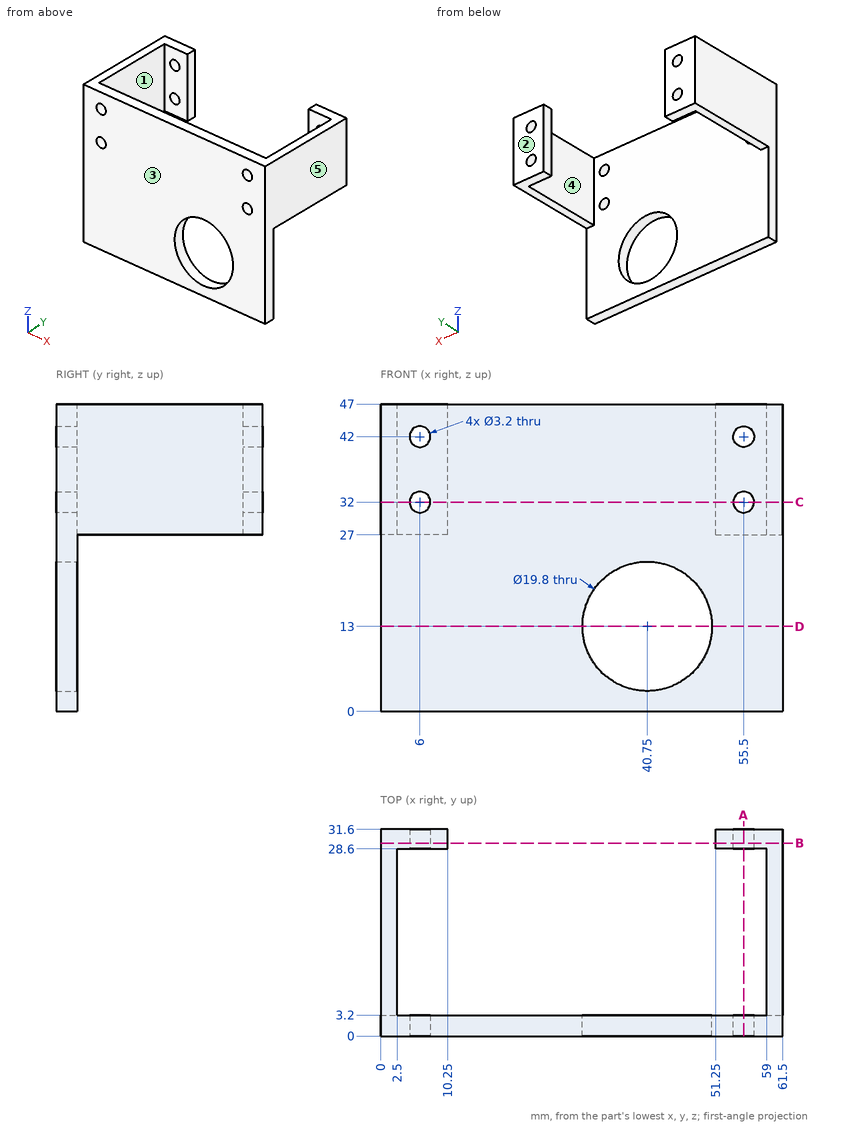
Source: three-view drawing plus pictorial views. Frame: mm from the lowest corner of the part. A direction names the side the tool comes from. Round coordinates to 2 decimals unless told otherwise and drop trailing zeros. Write each loop counter-clockwise with the first axis right and the second up, starting at its lowest first coordinate (ties: lowest second). Pieces come first, ordered by that corner, then holes. Notation, with made-up numbers: M -4.75,20.5 L 46.25,20.5 A25 cw 46.25,35.5 Z; hole C 42,23.25 d6. An arc over 180 degrees is marked long. Write item = value, one per line.
Item 1: Section query A-A on x = 55.5. Return loops of the section in (y, z), then the cut area to 3 significant figures.
Findings:
outline = M 0,0 L 3.2,0 L 3.2,30.4 L 0,30.4 Z; M 0,33.6 L 3.2,33.6 L 3.2,40.4 L 0,40.4 Z; M 0,43.6 L 3.2,43.6 L 3.2,47 L 0,47 Z; M 28.6,27 L 31.6,27 L 31.6,30.4 L 28.6,30.4 Z; M 28.6,33.6 L 31.6,33.6 L 31.6,40.4 L 28.6,40.4 Z; M 28.6,43.6 L 31.6,43.6 L 31.6,47 L 28.6,47 Z
area = 171 mm^2
Item 2: Access query for the marked faces 1 and 2. Directions: +Z, -Z, +X, -X, +Y, -Y. A direction counts if a zero-diameter tool reaches every point of the face in a straight line with its end or side. Return the directions, or none.
Findings:
face_1 = +Z, -Z
face_2 = +Z, -Z, +X, -X, +Y
Item 3: Section query B-B on y = 29.5. Return loops of the section in (x, z), then the cut area to 3 significant figures.
Findings:
outline = M 0,27 L 10.25,27 L 10.25,47 L 0,47 Z; M 51.25,27 L 61.5,27 L 61.5,47 L 51.25,47 Z; hole C 6,32 d3.2; hole C 6,42 d3.2; hole C 55.5,32 d3.2; hole C 55.5,42 d3.2
area = 378 mm^2
Item 4: Section query C-C on z = 32. Return loops of the section in (x, y), then the cut area to 3 significant figures.
Findings:
outline = M 0,0 L 4.4,0 L 4.4,3.2 L 2.5,3.2 L 2.5,28.6 L 4.4,28.6 L 4.4,31.6 L 0,31.6 Z; M 7.6,0 L 53.9,0 L 53.9,3.2 L 7.6,3.2 Z; M 7.6,28.6 L 10.25,28.6 L 10.25,31.6 L 7.6,31.6 Z; M 51.25,28.6 L 53.9,28.6 L 53.9,31.6 L 51.25,31.6 Z; M 57.1,0 L 61.5,0 L 61.5,31.6 L 57.1,31.6 L 57.1,28.6 L 59,28.6 L 59,3.2 L 57.1,3.2 Z
area = 346 mm^2
Item 5: Material intervals for line 1 along X through (y, z) = (1.9, 32); line 2 along X through (y, z) = (30.95, 42); line 3 along Z through (x, y) = (6, 30), sorted ascending. Write a range as [from, to].
Findings:
line_1 = [0, 4.4], [7.6, 53.9], [57.1, 61.5]
line_2 = [0, 4.4], [7.6, 10.25], [51.25, 53.9], [57.1, 61.5]
line_3 = [27, 30.4], [33.6, 40.4], [43.6, 47]
Item 6: Section query D-D on z = 13. Return loops of the section in (x, y).
Findings:
outline = M 0,0 L 30.85,0 L 30.85,3.2 L 0,3.2 Z; M 50.65,0 L 61.5,0 L 61.5,3.2 L 50.65,3.2 Z
Item 7: Pin query (flat end, axial travel): P1, Ø3, axis at y = 6, z = 8.5, coming from the -X side; P2, Ø23, axis at x = 40.75, z = 13, coming from the +Y side; P3, Ø8, axis at x = 58, y = 23.5, coming from the -Z side. Return the tip coordinate at first contact, or that it passes through.
Findings:
P1 = through
P2 = 3.2
P3 = 27
Item 8: Pull-direction query (X, two-part tool) for the marked faces 3, 4 and 5; classes: pulls with the +X half, pulls with the -X half, needs draft (parallel to the pull), parting line crosses it, or undercut.
Findings:
face_3 = needs draft
face_4 = undercut
face_5 = pulls with the +X half
